Geometry: final body of the model. Coordinates: model frame, mm. A direction names the side the tool comes from. Round coordinates to 2 decimals unless told otherwise and drop trailing zeros. Loops run counter-clockwise (first coordinate to the right, second up) from the corner with the lowest first, then second, coordinate; pieces in that order, holes last. Notation, with made-up numbers: M -23,54.25 L -9,54.25 A11 ccw -9,75.25 Z; hole C 80.5,-3 d1. An arc over 180 degrees is marked long. Return JSON: item names as keys, results as strings.
from build123d import *

# Parameters (mm, degrees)
SKETCH2_W                     = 63.3
SKETCH2_H                     = 30.32
BOSS_EXTRUDE1_DEPTH           = 5
SKETCH1_W                     = 40.64
SKETCH1_H                     = 20.32
SKETCH1_W_2                   = 2.38
SKETCH1_H_2                   = 6.35
CUT_EXTRUDE3_DEPTH            = 6
SKETCH3_W                     = 40.64
SKETCH3_H                     = 20.32
SKETCH3_W_2                   = 2.38
SKETCH3_H_2                   = 6.35
CUT_EXTRUDE5_DEPTH            = 6
SKETCH7_W                     = 63.3
SKETCH7_H                     = 30.32
BOSS_EXTRUDE2_DEPTH           = 2
SKETCH10_R                    = 2.78
BOSS_EXTRUDE3_DEPTH           = 10
SKETCH11_W                    = 63.3
SKETCH11_H                    = 30.32
BOSS_EXTRUDE4_DEPTH           = 2
SKETCH12_R                    = 2.78
BOSS_EXTRUDE5_DEPTH           = 10
FILLET1_R                     = 1
CSK_FOR_M3_SFHCS1_D           = 3.4
CSK_FOR_M3_SFHCS1_CSINK_D     = 6.72
CSK_FOR_M3_SFHCS1_CSINK_ANGLE = 90


with BuildPart() as part:
    # Sketch2 → Boss-Extrude1 (new body)
    with BuildSketch(Plane(origin=(0, 0, 0), x_dir=(0, 0, -1), z_dir=(1, 0, 0))):
        Rectangle(SKETCH2_W, SKETCH2_H)
        Polygon((181.65, 5), (31.65, 5), (31.65, 0), (31.65, -5), (181.65, -5), (181.65, 0), align=None)
        Polygon((181.65, 15.16), (181.65, 5), (181.65, 0), (181.65, -5), (181.65, -15.16), (244.95, -15.16), (244.95, 15.16), align=None)
    extrude(amount=BOSS_EXTRUDE1_DEPTH)

    # Sketch1 → Cut-Extrude3 (cut, through all)
    with BuildSketch(Plane(origin=(0, 0, 0), x_dir=(0, 0, -1), z_dir=(1, 0, 0))):
        Rectangle(SKETCH1_W, SKETCH1_H)
        with Locations((21.51, -0.015)):
            Rectangle(SKETCH1_W_2, SKETCH1_H_2)
    extrude(amount=CUT_EXTRUDE3_DEPTH, mode=Mode.SUBTRACT)

    # Sketch3 → Cut-Extrude5 (cut, through all)
    with BuildSketch(Plane(origin=(5, 0, 0), x_dir=(0, 0, -1), z_dir=(1, 0, 0))):
        with Locations((213.3, 0)):
            Rectangle(SKETCH3_W, SKETCH3_H)
        with Locations((234.81, 0)):
            Rectangle(SKETCH3_W_2, SKETCH3_H_2)
    extrude(amount=-CUT_EXTRUDE5_DEPTH, mode=Mode.SUBTRACT)

    # Sketch7 → Boss-Extrude2 (add)
    with BuildSketch(Plane(origin=(5, 0, 0), x_dir=(0, 0, -1), z_dir=(1, 0, 0))):
        Rectangle(SKETCH7_W, SKETCH7_H)
    extrude(amount=BOSS_EXTRUDE2_DEPTH)

    # Sketch10 → Boss-Extrude3 (add)
    with BuildSketch(Plane(origin=(7, 0, 0), x_dir=(0, 0, -1), z_dir=(1, 0, 0))):
        with Locations((10.12, 0)):
            Circle(SKETCH10_R)
    extrude(amount=BOSS_EXTRUDE3_DEPTH)

    # Sketch11 → Boss-Extrude4 (add)
    with BuildSketch(Plane(origin=(5, 0, 0), x_dir=(0, 0, -1), z_dir=(1, 0, 0))):
        with Locations((213.3, 0)):
            Rectangle(SKETCH11_W, SKETCH11_H)
    extrude(amount=BOSS_EXTRUDE4_DEPTH)

    # Sketch12 → Boss-Extrude5 (add)
    with BuildSketch(Plane(origin=(7, 0, 0), x_dir=(0, 0, -1), z_dir=(1, 0, 0))):
        with Locations((223.42, 0)):
            Circle(SKETCH12_R)
    extrude(amount=BOSS_EXTRUDE5_DEPTH)

    # Fillet1
    fillet1_edges = [part.edges().sort_by_distance(p)[0] for p in [
        (3.5, -15.16, -244.95),
        (3.5, 15.16, -244.95),
        (3.5, 15.16, -181.65),
        (2.5, 5, -181.65),
        (3.5, -15.16, -181.65),
        (2.5, -5, -181.65),
        (2.5, -5, -31.65),
        (2.5, 5, -31.65),
        (3.5, 15.16, -31.65),
        (3.5, -15.16, -31.65),
        (3.5, -15.16, 31.65),
        (3.5, 15.16, 31.65),
    ]]
    fillet(fillet1_edges, radius=FILLET1_R)

    # CSK for M3 SFHCS1 (through all)
    with Locations(Plane(origin=(7, 0, 0), x_dir=(0, 0, -1), z_dir=(1, 0, 0))):
        with Locations((-24.13, 5.08), (-24.13, -5.08), (24.13, -5.08), (24.13, 5.08), (189.17, 5.08), (189.17, -5.08), (237.43, 5.08), (237.43, -5.08)):
            CounterSinkHole(CSK_FOR_M3_SFHCS1_D / 2, CSK_FOR_M3_SFHCS1_CSINK_D / 2, counter_sink_angle=CSK_FOR_M3_SFHCS1_CSINK_ANGLE)


solid = part.part
Q1. Pull-direction query (Z, two-part tool) for faces 4 (the flat face through (3, 0, -244.95)), 5 (the flat face through (17, 0, -223)), 6 (the flat face through (2, 7, -20.32)); classes: pulls with the +Z half, pulls with the -Z half, needs draft (parallel to the pull), parting line crosses it, or undercut.
Determined:
{"face 4": "pulls with the -Z half", "face 5": "needs draft", "face 6": "undercut"}
Q2. Section query B-B (x = 10). Output: boundary loops of the cut face in (y, z), plus the area to 3 significant figures.
Determined:
{"outline": "C 0,-223.42 d5.56; C 0,-10.12 d5.56", "area": "48.6 mm^2"}
Q3. Material intervals for L1, parallel to Y at x = 1.55, z = -237.43; L2, parallel to Z at x = 2.25, y = 1; L3, parallel to Y at x = 4.5, z = -21.5, sorted ascending.
Determined:
{"L1": "y = -15.16 to -6.78, -3.38 to 3.38, 6.78 to 15.16", "L2": "z = -244.95 to -236, -192.98 to -22.7, 20.32 to 31.65", "L3": "y = -15.16 to -3.19, 3.16 to 15.16"}
Q4. Reachability of faces 1 (the cylindrical face through (11.93, -1.06, -12.69)), 2 (the flat face through (0, -1, -106)), 3 (the flat face through (2, 0, -22.7)) from +Z, -Z, +X, -X, +Y, -Y: full face, straight path, thin tool, end or side. Return the list, or none.
Determined:
{"face 1": "+X", "face 2": "+Z, -Z, -X, +Y, -Y", "face 3": "-X"}
Q5. Pin query (flat end, axial travel): pin 1 (10 mm diameter, centred on x = 2.5, z = -167.5, fed in from -Y); pin 2 (2 mm diameter, centred on x = 9, y = -8.5, fed in from -Z); pin 3 (6 mm diameter, centred on y = -0.5, z = -152, fed in from +X); pin 4 (10 mm diameter, centred on y = -11, z = -3.5, fed in from +X). Return the tip coordinate at first contact, or that it passes through.
Determined:
{"pin 1": "stops at y = -5", "pin 2": "passes through", "pin 3": "stops at x = 5", "pin 4": "stops at x = 7"}
Q6. Section query A-A (z = -213). Output: boundary loops of the cut face in (x, y).
Determined:
{"outline": "M 0,-15.16 L 7,-15.16 L 7,15.16 L 0,15.16 L 0,10.16 L 5,10.16 L 5,-10.16 L 0,-10.16 Z"}
